from build123d import *

# Parameters (mm, degrees)
F1_DEPTH = 35
F3_DEPTH = 25
F5_DEPTH = 8.5000004619
F6_D     = 6.5
F6_DEPTH = 5
F6_TIP   = 1.9527970118


with BuildPart() as f1:
    # F0 (on Top) → F1 (new body)
    with BuildSketch(Plane.XY):
        Polygon((72, 0), (0, 0), (0, 72), (-46.5, 72), (-46.5, -46.5), (0, -46.5), (72, -46.5), align=None)
    extrude(amount=F1_DEPTH)

    # F2 (on face) → F3 (cut)
    with BuildSketch(Plane.XY.offset(35)):
        Polygon((-41, 72), (-41, -41), (72, -41), (72, -5.5), (-5.5, -5.5), (-5.5, 72), align=None)
    extrude(amount=-F3_DEPTH, mode=Mode.SUBTRACT)

    # F4 (on face) → F5 (cut)
    with BuildSketch(Plane.XY.offset(10)):
        with BuildLine():
            Line((-14.2343885399, -14.2343885399), (-32.2656114601, -32.2656114601))
            ThreePointArc((-32.2656114601, -32.2656114601), (-18.3707862373, -35.0294640395), (-10.5, -23.25))
            ThreePointArc((-10.5, -23.25), (-11.4705359605, -18.3707862373), (-14.2343885399, -14.2343885399))
        make_face()
        with BuildLine():
            ThreePointArc((-14.2343885399, -14.2343885399), (-32.2656114601, -14.2343885399), (-32.2656114601, -32.2656114601))
            Line((-32.2656114601, -32.2656114601), (-14.2343885399, -14.2343885399))
        make_face()
    extrude(amount=-F5_DEPTH, mode=Mode.SUBTRACT)

    # F6
    with Locations(Plane.XY.offset(10)):
        with Locations((31.75, -23.25), (-23.25, 31.75)):
            Hole(F6_D / 2, depth=F6_DEPTH)
            with Locations((0, 0, -(F6_DEPTH + F6_TIP / 2))):  # 118° drill point
                Cone(0, F6_D / 2, F6_TIP, mode=Mode.SUBTRACT)


solid = f1.part
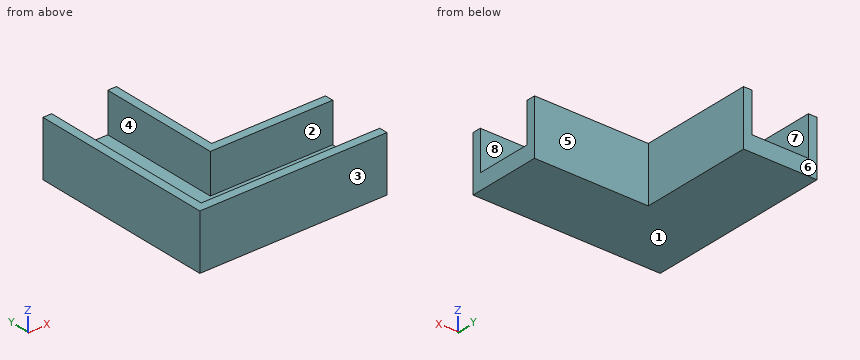
Here's how the part is built. I have some questions about the finished solid (model axes, mm). Face numbers are marked on the shaded views. A direction names the side the tool comes from. Coordinates: 2 decimals unless noted, no trailing zeros. Order: outer loops, then holes, each group sorted by start corner. A loop starts at its lowest first (then second) coordinate and runs counter-clockwise, first axis right, second up.
Item 1: If we mould it in two halves opening along Y, with no side actions, what happens to the marked faces 6, 7 and 8? For each: +Y half, -Y half, draft (parallel to the pull), parting line (faces both ways), or undercut.
Result sheet:
face 6: +Y half
face 7: draft
face 8: undercut
Item 2: I need wall thicknesses on line 1 (Y direction, x = -23.25, z = 7.55); line 2 (Y direction, x = 50.5, z = 30). Which ranges of each line are inside material? Lowest first, please.
Result sheet:
line 1: y = -46.5 to -36, -10.5 to 28.5, 35 to 72
line 2: y = -46.5 to -41, -5.5 to 0
Item 3: If we section it at C-C on y = -3: List the corners of the cut face in (x, z) for me.
Result sheet:
outline: (-46.5, 0) - (72, 0) - (72, 35) - (-5.5, 35) - (-5.5, 10) - (-41, 10) - (-41, 35) - (-46.5, 35) - close
Item 4: For the marked faces 1, 2, 3, 4 and 5, which set-ups out of +Z, -Z, +X, -X, +Y, -Y let a thin tool reach every point of the face, with its end or its side?
Result sheet:
face 1: -Z, +X, -X, +Y, -Y
face 2: +Z, +X
face 3: +Z, -Z, +X, -X, -Y
face 4: +Z, +Y
face 5: +Z, -Z, +X, +Y
Item 5: If we section it at D-D on z = 7: List the corners of the cut face in (x, y) for me.
Result sheet:
outline: (-46.5, -46.5) - (72, -46.5) - (72, 0) - (0, 0) - (0, 72) - (-46.5, 72) - close; hole circle Ø25.5 at (-23.25, -23.25); hole circle Ø6.5 at (-23.25, 31.75); hole circle Ø6.5 at (31.75, -23.25)
Item 6: If we section it at A-A on z = 29.5: List the corners of the cut face in (x, y) for me.
Result sheet:
outline: (-46.5, -46.5) - (72, -46.5) - (72, -41) - (-41, -41) - (-41, 72) - (-46.5, 72) - close; (-5.5, -5.5) - (72, -5.5) - (72, 0) - (0, 0) - (0, 72) - (-5.5, 72) - close
Item 7: If we section it at B-B on x = 10: List the corners of the cut face in (y, z) for me.
Result sheet:
outline: (-46.5, 0) - (0, 0) - (0, 35) - (-5.5, 35) - (-5.5, 10) - (-41, 10) - (-41, 35) - (-46.5, 35) - close
Item 8: For P1, Ø2, axis at y = 52, z = 17, coming from the +X side; P2, Ø17.5, axis at x = 20.5, z = 10.5, coming from the +Y side; P3, Ø8.5, axis at x = -23.25, y = 31.75, coming from the +Z side, each with a flat end and sliding along its axis, tell me the tip position at first contact or that it passes through.
Result sheet:
P1: stops at x = 0
P2: stops at y = 0
P3: stops at z = 10
